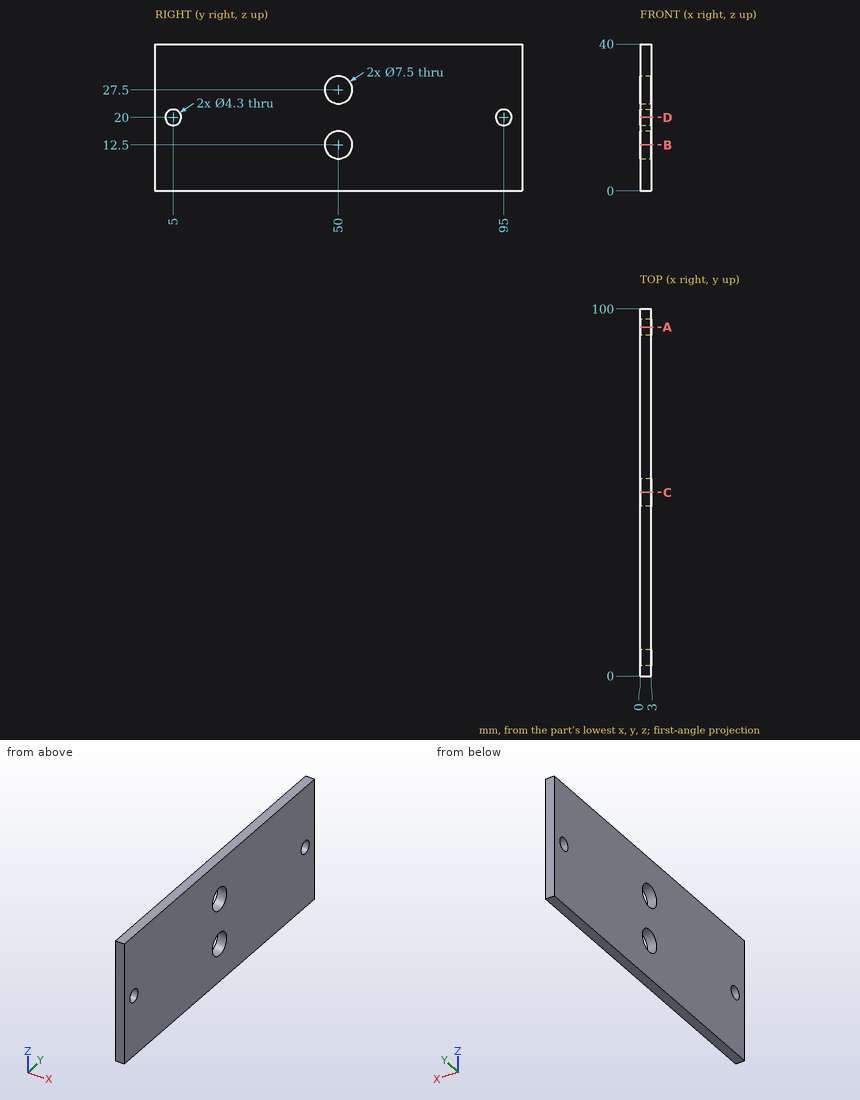
Geometry: see drawing. Coordinates: mm, zero at the bounding-box minimum. Round coordinates to 2 decimals unless told otherwise and drop trailing zeros. Write each loop counter-clockwise with the first axis right and the second up, starting at its lowest first coordinate (ties: lowest second). Pieces come first, ordered by that corner, then holes.
Item 1: Section query A-A (y = 95). Return loops of the section in (x, z), plus the area to 3 significant figures.
Item 2: Section query C-C (y = 50). Return loops of the section in (x, z), plus the area to 3 significant figures.
Item 3: Section query B-B (z = 12.5). Return loops of the section in (x, y), plus the area to 4 significant figures.
Item 4: Section query D-D (z = 20). Return loops of the section in (x, y).
Item 5: Material intervals for L1, parallel to Y at x = 2.4, z = 20; L2, parallel to Y at x = 0.65, z = 21.5; L3, parallel to Y at x = 2.15, z = 27.5, sorted ascending.
Completed:
1. outline: (0, 0) - (3, 0) - (3, 17.85) - (0, 17.85) - close; (0, 22.15) - (3, 22.15) - (3, 40) - (0, 40) - close
1. area: 107 mm2
2. outline: (0, 0) - (3, 0) - (3, 8.75) - (0, 8.75) - close; (0, 16.25) - (3, 16.25) - (3, 23.75) - (0, 23.75) - close; (0, 31.25) - (3, 31.25) - (3, 40) - (0, 40) - close
2. area: 75.0 mm2
3. outline: (0, 0) - (3, 0) - (3, 46.25) - (0, 46.25) - close; (0, 53.75) - (3, 53.75) - (3, 100) - (0, 100) - close
3. area: 277.5 mm2
4. outline: (0, 0) - (3, 0) - (3, 2.85) - (0, 2.85) - close; (0, 7.15) - (3, 7.15) - (3, 92.85) - (0, 92.85) - close; (0, 97.15) - (3, 97.15) - (3, 100) - (0, 100) - close
5. L1: y = 0 to 2.85, 7.15 to 92.85, 97.15 to 100
5. L2: y = 0 to 3.46, 6.54 to 93.46, 96.54 to 100
5. L3: y = 0 to 46.25, 53.75 to 100
